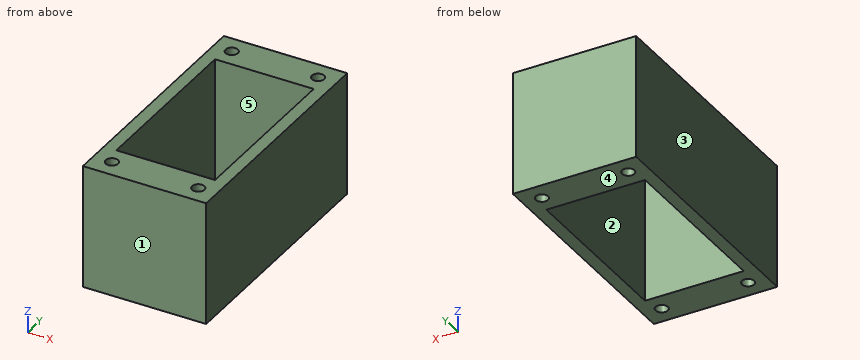
```python
from build123d import *

# Parameters (mm, degrees)
SKETCH1_W           = 50
SKETCH1_H           = 100
SKETCH1_R           = 2.5
BOSS_EXTRUDE1_DEPTH = 50
SKETCH2_W           = 40
SKETCH2_H           = 70
CUT_EXTRUDE1_DEPTH  = 93


with BuildPart() as part:
    # Sketch1 → Boss-Extrude1 (new body)
    with BuildSketch(Plane.XY):
        Rectangle(SKETCH1_W, SKETCH1_H)
        with Locations((-17.5, 42.5)):
            Circle(SKETCH1_R, mode=Mode.SUBTRACT)
        with Locations((17.5, 42.5)):
            Circle(SKETCH1_R, mode=Mode.SUBTRACT)
        with Locations((-17.5, -42.5)):
            Circle(SKETCH1_R, mode=Mode.SUBTRACT)
        with Locations((17.5, -42.5)):
            Circle(SKETCH1_R, mode=Mode.SUBTRACT)
    extrude(amount=BOSS_EXTRUDE1_DEPTH)

    # Sketch2 → Cut-Extrude1 (cut)
    with BuildSketch(Plane.XY.offset(50)):
        Rectangle(SKETCH2_W, SKETCH2_H)
    extrude(amount=-CUT_EXTRUDE1_DEPTH, mode=Mode.SUBTRACT)


solid = part.part
```
Model file for the job. Use its own axes, mm. Face numbers are marked on the shaded views. A direction names the side the tool comes from. Coordinates: 2 decimals unless noted, no trailing zeros. Write each loop counter-clockwise with the first axis right and the second up, starting at its lowest first coordinate (ties: lowest second). Pieces come first, ordered by that corner, then holes. Notation, with made-up numbers: (44, 87.5) - (58, 87.5) arc R13 cw to (58, 102.5) - close; hole circle Ø4 at (-40, 51). An arc over 180 degrees is marked (long way). One line per question, with ' | ' between items. Start each with the question number.
Q1. Cut at D-D, the plane y = 42.5. List the corners of the cut face in (x, z).
Q2. Cut at B-B, the plane x = -17.5. List the corners of the cut face in (y, z), then the cut area to 3 significant figures.
Q3. Pin check, flat tips, straight feed: pin 1 (3 mm diameter, centred on x = -17.5, y = 42.5, fed in from -Z); pin 2 (6.5 mm diameter, centred on x = 17.5, y = 42.5, fed in from -Z). Stop position of each tip, or through.
Q4. 3-axis set-ups, long thin cutter, end or side, ignore diameter. For the marked faces 4 and 5: which of +Z, -Z, +X, -X, +Y, -Y reach the whole face in a straight line?
Q5. Drill centre lines: line 1 (Y direction, x = -17.5, z = 38); line 2 (X direction, y = 23, z = 3.5); line 3 (Y direction, x = -8.5, z = 43). Where is each one in solid material? Low to high. Write a range as [from, to].
Q6. Cut at A-A, the plane y = -9. List the corners of the cut face in (x, z).
Q7. Pull direction Y, two halves, no side cores. Call the marked faces 1, 2 and 3: pulls with the +Y half, pulls with the -Y half, needs draft (parallel to the pull), parting line crosses it, or undercut.
Q8. Cut at C-C, the plane x = -12. List the corners of the cut face in (y, z), then the cut area to 3 significant figures.
Answer below:
1) outline: (-25, 0) - (-20, 0) - (-20, 50) - (-25, 50) - close; (-15, 0) - (15, 0) - (15, 50) - (-15, 50) - close; (20, 0) - (25, 0) - (25, 50) - (20, 50) - close
2) outline: (-50, 0) - (-45, 0) - (-45, 50) - (-50, 50) - close; (-40, 0) - (-35, 0) - (-35, 50) - (-40, 50) - close; (35, 0) - (40, 0) - (40, 50) - (35, 50) - close; (45, 0) - (50, 0) - (50, 50) - (45, 50) - close | area: 1,000 mm^2
3) pin 1: through | pin 2: z = 0
4) face 4: -Z, +X, -X, +Y, -Y | face 5: +Z, -Z
5) line 1: [-50, -45], [-40, -35], [35, 40], [45, 50] | line 2: [-25, -20], [20, 25] | line 3: [-50, -35], [35, 50]
6) outline: (-25, 0) - (-20, 0) - (-20, 50) - (-25, 50) - close; (20, 0) - (25, 0) - (25, 50) - (20, 50) - close
7) face 1: pulls with the -Y half | face 2: undercut | face 3: needs draft
8) outline: (-50, 0) - (-35, 0) - (-35, 50) - (-50, 50) - close; (35, 0) - (50, 0) - (50, 50) - (35, 50) - close | area: 1,500 mm^2
